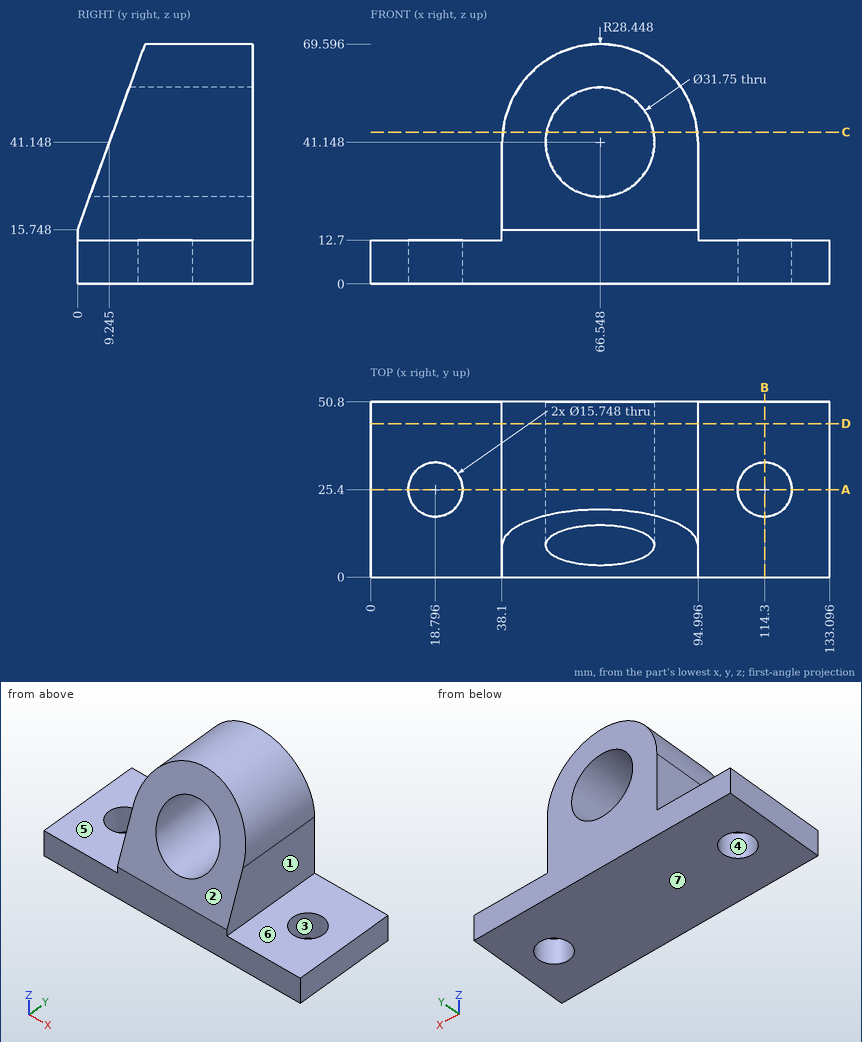
The drawing under review shows one solid part. Ordinate dimensions are in mm from its lowest x, y, z. A direction names the side the tool comes from. Round coordinates to 2 decimals unless told otherwise and drop trailing zeros. Loops run counter-clockwise (first coordinate to the right, second up) from the corner with the lowest first, then second, coordinate; pieces in that order, holes last.
Item 1: Mouldability with a two-part tool opening along Y and no side actions: class the marked faces 1, 2, 3 and 4 as released by +Y, released by -Y, zero draft, split by the parting line, or undercut.
Determined:
face 1: zero draft
face 2: released by -Y
face 3: undercut
face 4: undercut
Item 2: Take a section at B-B (x = 114.3). Write out the cut boundary in (y, z), then the cut area to 3 significant figures.
Determined:
outline: (0, 0) - (17.53, 0) - (17.53, 12.7) - (0, 12.7) - close; (33.27, 0) - (50.8, 0) - (50.8, 12.7) - (33.27, 12.7) - close
area: 445 mm2
Item 3: Take a section at A-A (y = 25.4). Write out the cut boundary in (x, z) (3 decimals).
Determined:
outline: (0, 0) - (10.922, 0) - (10.922, 12.7) - (0, 12.7) - close; (26.67, 0) - (106.426, 0) - (106.426, 12.7) - (94.996, 12.7) - (94.996, 41.148) arc R28.448 ccw to (38.1, 41.148) - (38.1, 12.7) - (26.67, 12.7) - close; (122.174, 0) - (133.096, 0) - (133.096, 12.7) - (122.174, 12.7) - close; hole circle Ø31.75 at (66.548, 41.148)
Item 4: Take a section at D-D (y = 44.5). Write out the cut boundary in (x, z) (3 decimals).
Determined:
outline: (0, 0) - (133.096, 0) - (133.096, 12.7) - (94.996, 12.7) - (94.996, 41.148) arc R28.448 ccw to (38.1, 41.148) - (38.1, 12.7) - (0, 12.7) - close; hole circle Ø31.75 at (66.548, 41.148)
Item 5: Clearance check with flat-ended pins moving along their axes: pin 1 Ø25 at (x, y) = (114.3, 25.4) entering from +Z; pin 2 Ø8.5 at (y, z) = (28.5, 20) entering from -X; pin 3 Ø8 at (x, y) = (14.5, 30.5) entering from -Z; pin 4 Ø1.5 at (y, z) = (44, 15.5) entering from +X. State where each tip first meets the part, or that it passes through.
Determined:
pin 1: stops at z = 12.7
pin 2: stops at x = 38.1
pin 3: stops at z = 0
pin 4: stops at x = 95
Item 6: Take a section at C-C (z = 44). Write out the cut boundary in (x, y) (1 decimal), then the cut area to 3 significant figures.
Determined:
outline: (38.2, 10.3) - (50.9, 10.3) - (50.9, 50.8) - (38.2, 50.8) - close; (82.2, 10.3) - (94.9, 10.3) - (94.9, 50.8) - (82.2, 50.8) - close
area: 1,030 mm2
Item 7: For line 1 (X direction, y = 25.4, z = 3.75); line 2 (X direction, y = 23, z = 8.5) (1 decimal); line 3 (Z direction, x = 125, y = 4.5), list the stretches that pass through material, from the lowest coordinate up.
Determined:
line 1: x = 0 to 10.92, 26.67 to 106.43, 122.17 to 133.1
line 2: x = 0 to 11.3, 26.3 to 106.8, 121.8 to 133.1
line 3: z = 0 to 12.7
Item 8: For the marked faces 5, 6 and 7, list the 3-axis set-ups (+Z, -Z, +X, -X, +Y, -Y) from which the entire face can be reached by the end or side of a thin tool; tool diameter is ignored.
Determined:
face 5: +Z, -X, +Y, -Y
face 6: +Z, +X, +Y, -Y
face 7: -Z, +X, -X, +Y, -Y
